Part print with two shaded views. Sizes in mm from the minimum x, y, z corner. Coordinates: 2 decimals unless noted, no trailing zeros. Order: outer loops, then holes, each group sorted by start corner. A loop starts at its lowest first (then second) coordinate and runs counter-clockwise, first axis right, second up.
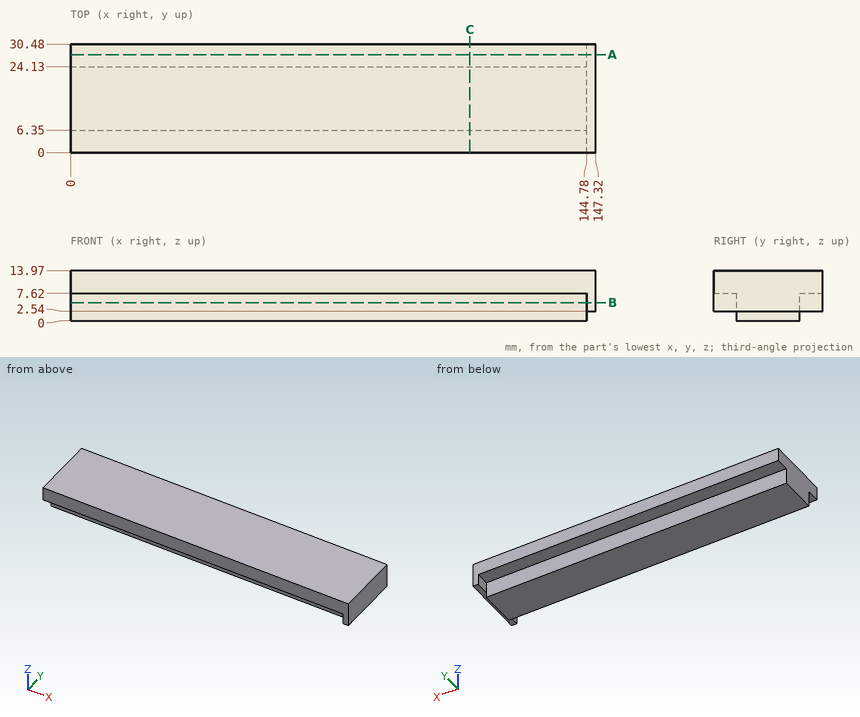
Q1. Cut at C-C on x = 112. Write the cut outline in (y, z).
Results list:
outline: (0, 7.62) - (6.35, 7.62) - (6.35, 0) - (24.13, 0) - (24.13, 7.62) - (30.48, 7.62) - (30.48, 13.97) - (0, 13.97) - close
Q2. Cut at B-B on z = 5. Write the cut outline in (x, y), and give its area (3 significant figures).
Results list:
outline: (0, 6.35) - (144.78, 6.35) - (144.78, 0) - (147.32, 0) - (147.32, 30.48) - (144.78, 30.48) - (144.78, 24.13) - (0, 24.13) - close
area: 2,650 mm2
Q3. Cut at A-A on y = 27.5. Write the cut outline in (x, z), and give its area (3 significant figures).
Results list:
outline: (0, 7.62) - (144.78, 7.62) - (144.78, 2.54) - (147.32, 2.54) - (147.32, 13.97) - (0, 13.97) - close
area: 948 mm2
Q4. Pin check, flat tips, straight feed: pin 1 Ø2.5 at (x, z) = (52, 5) entering from -Y; pin 2 Ø2 at (y, z) = (19.5, 1.5) entering from +X; pin 3 Ø6 at (x, z) = (75, 2.5) entering from +Y. Stop position of each tip, or through.
Results list:
pin 1: stops at y = 6.35
pin 2: stops at x = 144.78
pin 3: stops at y = 24.13
Q5. Wall check: line 1 along Y through (x, z) = (27, 2.5); line 2 along X through (y, z) = (6, 5.5); line 3 along Z through (x, y) = (18.5, 5). Give the ranges that are in metal, low to high.
Results list:
line 1: y = 6.35 to 24.13
line 2: x = 144.78 to 147.32
line 3: z = 7.62 to 13.97
